Verification items for the finished model (mm, model axes). A direction names the side the tool comes from. Round coordinates to 2 decimals unless told otherwise and drop trailing zeros. Order: outer loops, then holes, each group sorted by start corner. A loop starts at its lowest first (then second) coordinate and runs counter-clockwise, first axis right, second up. Notation, with made-up numbers: M 36.25,82.5 L 51.25,82.5 A34 ccw 51.25,116.5 Z; hole C 36.25,-9.75 d8. An arc over 180 degrees is marked long. Use CSV: the item, a comma, the result in double quotes. Start each with the question number.
Q1. Scan lines: line 1 (Z direction, x = 41, y = 81); line 2 (X direction, y = 47, z = 22). Record each from-to range of solid material in increasing order.
Q2. Sectioned sample at A-A (y = 52). Enter the section's corners in (x, z), and give its area (3 significant figures).
Q3. Mould release check, pull along Z, two halves, no side actions. Record for faces 3 (the face through (146.05, 27, 77)), 4 (the face through (58, 40, 152.4)), 5 (the face through (75, 0, 75)): +Z half, -Z half, draft (parallel to the pull), parting line (faces both ways), or undercut.
Q4. Sectioned sample at B-B (y = 22). Enter the section's corners in (x, z), and give its area (3 significant figures).
Q5. Set-up check for faces 1 (the face through (6, 101.6, 59)), 2 (the face through (60, 48, 146.05)): record each of +Z, -Z, +X, -X, +Y, -Y from which the full face is reachable in a straight line by a thin tool's end or side.
Q6. Sectioned sample at C-C (z = 119.5). Enter the section's corners in (x, y), and give its area (3 significant figures).
Q7. Gauge pin test, flat end, axial feed: pin 1 Ø10 at (y, z) = (73.5, 87) entering from +X. Record the tip position at first contact, or that the pin passes through.
```python
from build123d import *

# Parameters (mm, degrees)
SKETCH1_W           = 152.4
SKETCH1_H           = 101.6
BOSS_EXTRUDE1_DEPTH = 152.4
CUT_EXTRUDE2_DEPTH  = 152.4
SKETCH7_W           = 139.7
SKETCH7_H           = 139.7
CUT_EXTRUDE3_DEPTH  = 88.9


with BuildPart() as part:
    # Sketch1 → Boss-Extrude1 (new body)
    with BuildSketch(Plane.XY):
        with Locations((76.2, 50.8)):
            Rectangle(SKETCH1_W, SKETCH1_H)
    extrude(amount=BOSS_EXTRUDE1_DEPTH)

    # Sketch6 → Cut-Extrude2 (cut)
    with BuildSketch(Plane.XY.offset(152.4)):
        Polygon((104.436678767, 101.6), (38.1, 101.6), (152.4, 38.1), (152.4, 101.6), (104.590197544, 101.6), align=None)
    extrude(amount=-CUT_EXTRUDE2_DEPTH, mode=Mode.SUBTRACT)

    # Sketch7 → Cut-Extrude3 (cut)
    with BuildSketch(Plane(origin=(0, 101.6, 0), x_dir=(1, 0, 0), z_dir=(0, 1, 0))):
        with Locations((76.2, -76.2)):
            Rectangle(SKETCH7_W, SKETCH7_H)
    extrude(amount=-CUT_EXTRUDE3_DEPTH, mode=Mode.SUBTRACT)


solid = part.part
```
Verdict:
1,line 1,"z = 0 to 6.35, 146.05 to 152.4"
1,line 2,"x = 0 to 6.35"
2,outline,"M 0,0 L 127.38,0 L 127.38,6.35 L 6.35,6.35 L 6.35,146.05 L 127.38,146.05 L 127.38,152.4 L 0,152.4 Z"
2,area,"2,500 mm²"
3,face 3,"undercut"
3,face 4,"+Z half"
3,face 5,"draft"
4,outline,"M 0,0 L 152.4,0 L 152.4,152.4 L 0,152.4 Z; hole M 6.35,6.35 L 146.05,6.35 L 146.05,146.05 L 6.35,146.05 Z"
4,area,"3,710 mm²"
5,face 1,"+Z, -Z, +X, -X, +Y"
5,face 2,"+Y"
6,outline,"M 0,0 L 152.4,0 L 152.4,38.1 L 146.05,41.63 L 146.05,12.7 L 6.35,12.7 L 6.35,101.6 L 0,101.6 Z"
6,area,"2,670 mm²"
7,pin 1,"stops at x = 6.35"
